Could you check a few things on this model? Use its own coordinates, in mm. A direction names the side the tool comes from. Round coordinates to 2 decimals unless told otherwise and drop trailing zeros. Loops run counter-clockwise (first coordinate to the right, second up) from the corner with the lowest first, then second, coordinate; pieces in that order, holes last. Notation, with made-up numbers: (-37, 38) -> (-28, 38) arc R14 ccw to (-28, 48) -> close; hole circle Ø6 at (23.25, 55.25). An arc over 180 degrees is marked (long way). Put each result on its own line as item: value. Start each with the question number.
1. Imagine slicing it at A-A, the plane x = -5.5. Please give me the cut outline in (y, z), and give its area (3 significant figures).
2. Which directions (+Z, -Z, +X, -X, +Y, -Y) give clear straight access to the entire face, cutting with the end or side of a thin tool? Please do faces 4 (the flat face through (69, 3, 58)), 5 (the flat face through (23, 3, 72)), 6 (the flat face through (-23, 3, -72)), 7 (the flat face through (69, 3, 0)), 8 (the flat face through (69, 3, -57)).
3. If we mould it in two halves opening along Z, with no side actions, what happens to faces 1 (the flat face through (-69, 3, 0)), 2 (the flat face through (-23, 3, 72)), 3 (the flat face through (58, 3, -69))? For each: pulls with the +Z half, pulls with the -Z half, needs draft (parallel to the pull), parting line crosses it, or undercut.
4. Imagine slicing it at B-B, the plane z = -56.5. Please give me the cut outline in (x, y), and give its area (3 significant figures).
5. I need wall thicknesses on line 1 (X direction, y = 2.35, z = 18). Which ranges of the line are inside material? Lowest first, please. Write a range as [from, to].
6. I'm going to push flat-ended pins straight in: P1, Ø12, axis at x = 31, z = -42.5, coming from the -Y side; P2, Ø3, axis at y = 4.5, z = 72, coming from the -X side; P3, Ø1.8, axis at y = 2.5, z = -72.5, coming from the +X side; P4, Ø1.8, axis at x = 2.5, y = 4, coming from the +Z side. Where does each tip first touch, or does it pass through?
```python
from build123d import *

# Parameters (mm, degrees)
BOSS_EXTRUDE1_DEPTH = 6


with BuildPart() as part:
    # Sketch1 → Boss-Extrude1 (new body)
    with BuildSketch(Plane(origin=(0, 0, 0), x_dir=(1, 0, 0), z_dir=(0, 1, 0))):
        Polygon((0, 69), (-23, 69), (-23, 75), (-46, 75), (-46, 69), (-69, 69), (-69, 46), (-75, 46), (-75, 23), (-69, 23), (-69, 0), (-69, -23), (-75, -23), (-75, -46), (-69, -46), (-69, -69), (-46, -69), (-46, -75), (-23, -75), (-23, -69), (0, -69), (23, -69), (23, -75), (46, -75), (46, -69), (69, -69), (69, -46), (75, -46), (75, -23), (69, -23), (69, 0), (69, 23), (75, 23), (75, 46), (69, 46), (69, 69), (46, 69), (46, 75), (23, 75), (23, 69), align=None)
    extrude(amount=BOSS_EXTRUDE1_DEPTH)


solid = part.part
```
Entries:
1. outline: (0, -69) -> (6, -69) -> (6, 69) -> (0, 69) -> close
1. area: 828 mm^2
2. face 4: +Z, +X, +Y, -Y
2. face 5: +Z, +Y, -Y
2. face 6: -Z, +Y, -Y
2. face 7: +X, +Y, -Y
2. face 8: -Z, +X, +Y, -Y
3. face 1: undercut
3. face 2: needs draft
3. face 3: pulls with the -Z half
4. outline: (-69, 0) -> (69, 0) -> (69, 6) -> (-69, 6) -> close
4. area: 828 mm^2
5. line 1: [-69, 69]
6. P1: y = 0
6. P2: x = -46
6. P3: x = 46
6. P4: z = 69
